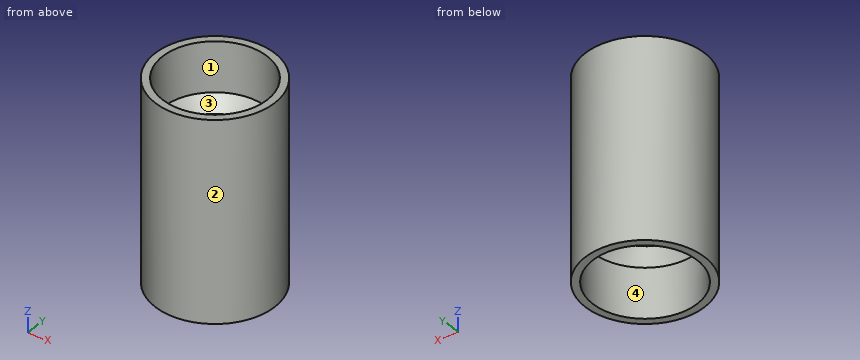
Solid Edge part; units mm, degrees
sketch "Sketch1" plane through (0, 0, 0) normal (0, -1, 0) x (1, 0, 0)
  line L0 (3, 11) -> (4.2, 11)
  line L1 (4.2, 11) -> (4.2, 16)
  line L2 (4.2, 16) -> (4.8, 16)
  line L3 (4.8, 16) -> (4.8, 0)
  line L4 (4.8, 0) -> (4.2, 0)
  line L5 (4.2, 0) -> (4.2, 5)
  line L6 (4.2, 5) -> (3, 5)
  line L7 (3, 5) -> (3, 11)
revolve "RevolvedProtrusion1" add sketch "Sketch1" angle 360 about axis through (0, 0, 0.6598) along (0, 0, 1)
chamfer "Chamfer1" distance 1 angle 45 2 edges at (-4.2, 0, 5) (-4.2, 0, 11)
Source: CAD feature listing. Evaluate the final solid. Frame: model axes, mm. Face numbers are marked on the shaded views. A direction names the side the tool comes from. Coordinates: 2 decimals unless noted, no trailing zeros. Loops run counter-clockwise (first coordinate to the right, second up) from the corner with the lowest first, then second, coordinate; pieces in that order, holes last. Notation, with made-up numbers: M 65.25,54.25 L 81.25,54.25 A22 ccw 81.25,61.25 Z; hole C 45,8.5 d9. An arc over 180 degrees is marked long. Answer in a Markdown table with one row per item.
Q1. Draft query along Y for the marked faces 1 and 2. Return one class per face: pulls with the +Y half, pulls with the -Y half, needs draft (parallel to the pull), parting line crosses it, or undercut.
Answers below:
| item | result |
|---|---|
| face 1 | undercut |
| face 2 | parting line crosses it |
Q2. Set-up query: the marked faces 3 and 4. Return all of +Z, -Z, +X, -X, +Y, -Y with unobstructed straight access to the full face (end or side cutting, diameter ignored); none if empty.
Answers below:
| item | result |
|---|---|
| face 3 | +Z |
| face 4 | -Z |
Q3. Section A-A on y = 0. Return the cut outline in (x, z).
Answers below:
| item | result |
|---|---|
| outline | M -4.8,0 L -4.2,0 L -4.2,4 L -3.2,5 L -3,5 L -3,11 L -3.2,11 L -4.2,12 L -4.2,16 L -4.8,16 Z; M 3,5 L 3.2,5 L 4.2,4 L 4.2,0 L 4.8,0 L 4.8,16 L 4.2,16 L 4.2,12 L 3.2,11 L 3,11 Z |
Q4. Section C-C on z = 3. Return the cut outline in (x, y).
Answers below:
| item | result |
|---|---|
| outline | C 0,0 d9.6; hole C 0,0 d8.4 |
Q5. Section D-D on z = 8.25. Return the cut outline in (x, y).
Answers below:
| item | result |
|---|---|
| outline | C 0,0 d9.6; hole C 0,0 d6 |
Q6. Ray query, probe 1 along Y at (x, z) = (0, 5.75); probe 2 along Y at (x, z) = (0, 2.7); probe 3 along Z at (x, y) = (-3, 1). Return the intervals inside material, ascending. Write a range as from..to.
Answers below:
| item | result |
|---|---|
| probe 1 | y = -4.8..-3, 3..4.8 |
| probe 2 | y = -4.8..-4.2, 4.2..4.8 |
| probe 3 | z = 5..11 |
Q7. First-contact query: pin 1 (1.9 mm diameter, centred on x = -1.5, y = -1, fed in from +Z); pin 2 (5 mm diameter, centred on x = 3.5, z = 11.5, fed in from +Y); pin 3 (5 mm diameter, centred on x = 3.5, z = 8, fed in from -Y). Flat tips, straight axial feed; report the tip coordinate or a pass-through.
Answers below:
| item | result |
|---|---|
| pin 1 | passes through |
| pin 2 | stops at y = 4.69 |
| pin 3 | stops at y = -4.69 |
